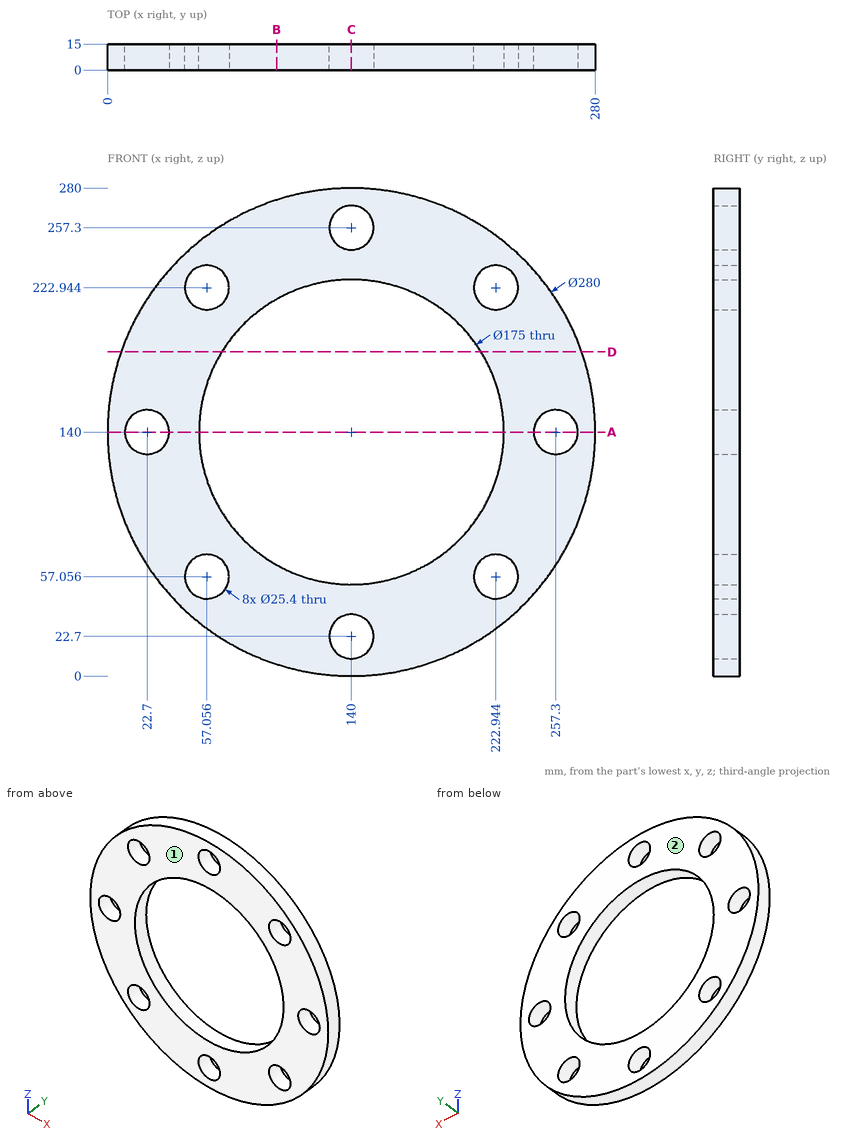
Drawing for the job (mm, zero at the part's lowest x, y, z). Give positions to 0.01 mm unless a question says otherwise; leave off trailing zeros. Loops run counter-clockwise (first coordinate to the right, second up) from the corner with the lowest first, then second, coordinate; pieces in that order, holes last.
Item 1: Slice it at A-A (z = 140). Write the cut outline in (x, y), plus the area to 3 significant figures.
Check values:
outline: (0, 0) - (10, 0) - (10, 15) - (0, 15) - close; (35.4, 0) - (52.5, 0) - (52.5, 15) - (35.4, 15) - close; (227.5, 0) - (244.6, 0) - (244.6, 15) - (227.5, 15) - close; (270, 0) - (280, 0) - (280, 15) - (270, 15) - close
area: 813 mm2
Item 2: Slice it at B-B (x = 97). Write the cut outline in (y, z) (1 decimal).
Check values:
outline: (0, 6.8) - (15, 6.8) - (15, 63.8) - (0, 63.8) - close; (0, 216.2) - (15, 216.2) - (15, 273.2) - (0, 273.2) - close
Item 3: Mould opens along Y. For the marked faces 1 and 2 say: +Y half, -Y half, draft (parallel to the pull), parting line (faces both ways), or undercut.
Check values:
face 1: -Y half
face 2: +Y half
Item 4: Drill centre lines: line 1 along Z through (x, y) = (140, 9.5); line 2 along X through (y, z) = (13.5, 139.5); line 3 along Z through (x, y) = (22.7, 4.75) (1 decimal). Where is each one in solid material? Low to high.
Check values:
line 1: z = 0 to 10, 35.4 to 52.5, 227.5 to 244.6, 270 to 280
line 2: x = 0 to 10.01, 35.39 to 52.5, 227.5 to 244.61, 269.99 to 280
line 3: z = 63.6 to 127.3, 152.7 to 216.4
Item 5: Slice it at C-C (x = 140). Write the cut outline in (y, z), plus the area to 3 significant figures.
Check values:
outline: (0, 0) - (15, 0) - (15, 10) - (0, 10) - close; (0, 35.4) - (15, 35.4) - (15, 52.5) - (0, 52.5) - close; (0, 227.5) - (15, 227.5) - (15, 244.6) - (0, 244.6) - close; (0, 270) - (15, 270) - (15, 280) - (0, 280) - close
area: 813 mm2
Item 6: Drop flat-ended pins along their axis: P1, Ø20.5, axis at x = 22.7, z = 140, coming from the +Y side; P2, Ø3, axis at x = 77, y = 12, coming from the -Z side; P3, Ø1, axis at x = 210.5, y = 3.5, coming from the +Z side; P4, Ø3, axis at x = 219.5, y = 1.5, coming from the -Z side. Give the stop position or say it passes through.
Check values:
P1: passes through
P2: stops at z = 14.23
P3: stops at z = 261.24
P4: stops at z = 23.74
Item 7: Slice it at D-D (z = 186). Write the cut outline in (x, y).
Check values:
outline: (7.77, 0) - (65.57, 0) - (65.57, 15) - (7.77, 15) - close; (214.43, 0) - (272.23, 0) - (272.23, 15) - (214.43, 15) - close
